The model under review builds one solid part; all positions refer to its coordinate system, in mm. Face numbers are marked on the shaded views. A direction names the side the tool comes from. Coordinates: 2 decimals unless noted, no trailing zeros. Loops run counter-clockwise (first coordinate to the right, second up) from the corner with the lowest first, then second, coordinate; pieces in that order, holes last. Notation, with made-up numbers: M 58.5,68 L 95.5,68 A7 cw 95.5,80 Z; hole C 17.25,44 d2. An arc over 180 degrees is marked long. One line per item, written item: value.
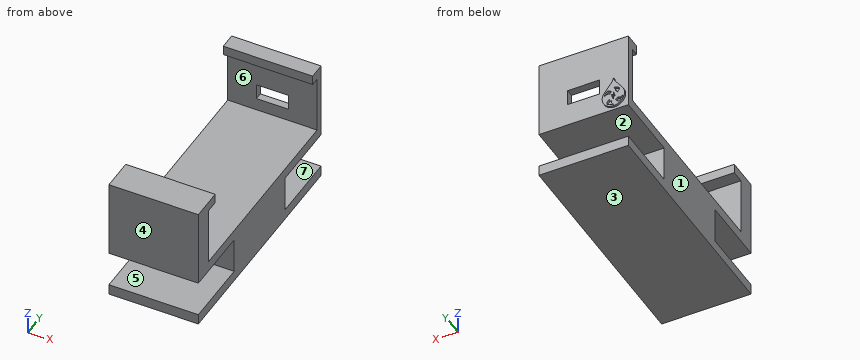
```python
from build123d import *

# Parameters (mm, degrees)
F0_W      = 42
F0_H      = 109.5
F1_DEPTH  = 5
F2_W      = 42
F2_H      = 7.5
F2_H_2    = 15
F3_DEPTH  = 32
F4_W      = 42
F4_H      = 27.5
F5_DEPTH  = 4
F6_W      = 42
F6_H      = 27.5
F7_DEPTH  = 6
F8_W      = 15
F8_H      = 7.5
F9_DEPTH  = 3.501
F10_W     = 42
F10_H     = 54.75
F11_DEPTH = 22
F12_W     = 42
F12_H     = 17
F13_DEPTH = 32
F14_W     = 42
F14_H     = 17
F15_DEPTH = 32
F17_DEPTH = 1


# Not quite as in the source:
# - a feature names something its author has since deleted; it is built from what else it names


with BuildPart() as f1:
    # F0 (on Top) → F1 (new body)
    with BuildSketch(Plane.XY):
        Rectangle(F0_W, F0_H)
    extrude(amount=F1_DEPTH)

    # F2 (on face) → F3 (join)
    with BuildSketch(Plane.XY.offset(5)):
        with Locations((0, 51)):
            Rectangle(F2_W, F2_H)
        with Locations((0, -47.25)):
            Rectangle(F2_W, F2_H_2)
    extrude(amount=F3_DEPTH)

    # F4 (on face) → F5 (cut)
    with BuildSketch(Plane.XZ.offset(-47.25)):
        with Locations((0, 18.75)):
            Rectangle(F4_W, F4_H)
    extrude(amount=-F5_DEPTH, mode=Mode.SUBTRACT)

    # F6 (on face) → F7 (cut)
    with BuildSketch(Plane(origin=(0, -39.75, 0), x_dir=(-1, 0, 0), z_dir=(0, 1, 0))):
        with Locations((0, 18.75)):
            Rectangle(F6_W, F6_H)
    extrude(amount=-F7_DEPTH, mode=Mode.SUBTRACT)

    # F8 (on face) → F9 (cut, through all)
    with BuildSketch(Plane.XZ.offset(-51.25)):
        with Locations((0, 14.75)):
            Rectangle(F8_W, F8_H)
    extrude(amount=-F9_DEPTH, mode=Mode.SUBTRACT)

    # F10 (on face) → F11 (join)
    with BuildSketch(Plane(origin=(0, 0, 0), x_dir=(1, 0, 0), z_dir=(0, 0, -1))):
        with Locations((0, -27.375)):
            Rectangle(F10_W, F10_H)
        with Locations((0, 27.375)):
            Rectangle(F10_W, F10_H)
    extrude(amount=F11_DEPTH)

    # F12 (on face) → F13 (cut)
    with BuildSketch(Plane(origin=(0, 54.75, 0), x_dir=(-1, 0, 0), z_dir=(0, 1, 0))):
        with Locations((0, -8.5)):
            Rectangle(F12_W, F12_H)
    extrude(amount=-F13_DEPTH, mode=Mode.SUBTRACT)

    # F14 (on face) → F15 (cut)
    with BuildSketch(Plane.XZ.offset(54.75)):
        with Locations((0, -8.5)):
            Rectangle(F14_W, F14_H)
    extrude(amount=-F15_DEPTH, mode=Mode.SUBTRACT)

    # F16 (on face) → F17 (join)
    with BuildSketch(Plane(origin=(0, 54.75, 0), x_dir=(-1, 0, 0), z_dir=(0, 1, 0))):
        with BuildLine():
            ThreePointArc((9.9006995692, 9.0004714316), (13.1670561221, 1.352687349), (19.7461517383, 6.4392566621))
            ThreePointArc((19.7461517383, 6.4392566621), (19.5019885984, 8.0225954525), (18.7921845523, 9.458825093))
            ThreePointArc((18.7921845523, 9.458825093), (14.575302704, 11.6944347601), (10.2883124178, 9.5963982037))
            add(Edge.make_bspline(
                [(9.9006995692, 9.0004714316), (10.0318943543, 9.2081460376), (10.1611439812, 9.4065291941), (10.2883124178, 9.5963982037)],
                knots=[0, 0, 0, 0, 0.0231761706, 0.0231761706, 0.0231761706, 0.0231761706], degree=3))
        make_face()
        with BuildLine():
            add(Edge.make_bspline(
                [(12.5148005536, 5.2476986911), (11.5117744305, 4.2282460665), (10.7037792288, 2.9078259209), (13.5031697151, 2.0462179781), (14.5618504929, 1.8354499162)],
                knots=[0, 0, 0, 0, 0.4579310006, 1, 1, 1, 1], degree=3))
            add(Edge.make_bspline(
                [(13.5659415486, 4.241716412), (12.8136013619, 4.2865276682), (12.6872834074, 4.7459304754), (12.5148005536, 5.2476986911)],
                knots=[0, 0, 0, 0, 1.4549562665, 1.4549562665, 1.4549562665, 1.4549562665], degree=3))
            add(Edge.make_bspline(
                [(14.5618504929, 1.8354499162), (14.5289066888, 1.9808173354), (13.3458541311, 2.6761364671), (13.5659415486, 4.241716412)],
                knots=[0, 0, 0, 0, 2.604218323, 2.604218323, 2.604218323, 2.604218323], degree=3))
        make_face(mode=Mode.SUBTRACT)
        Polygon((13.47238521, 7.6377728132), (14.4902859979, 7.2816363839), (14.4902859979, 9.0213598503), (15.3866174204, 5.9906424503), (14.4902859979, 6.4392566621), (14.4902859979, 4.5215808953), align=None, mode=Mode.SUBTRACT)
        with BuildLine():
            add(Edge.make_bspline(
                [(15.4229601255, 4.1801771125), (16.5064311467, 3.1538456327), (16.8590547707, 1.9119603138), (18.5636819849, 4.2745726241), (19.0433704887, 5.2473602224)],
                knots=[0, 0, 0, 0, 0.4553347248, 1, 1, 1, 1], degree=3))
            add(Edge.make_bspline(
                [(16.4662250147, 5.1379367456), (16.2283618655, 4.4227829667), (15.8584250881, 4.3158873473), (15.4229601255, 4.1801771125)],
                knots=[0, 0, 0, 0, 1.4162291989, 1.4162291989, 1.4162291989, 1.4162291989], degree=3))
            add(Edge.make_bspline(
                [(19.0433704887, 5.2473602224), (18.3244173567, 4.9723164216), (17.3367887913, 4.1913386793), (16.4662250147, 5.1379367456)],
                knots=[0, 0, 0, 0, 2.5794674433, 2.5794674433, 2.5794674433, 2.5794674433], degree=3))
        make_face(mode=Mode.SUBTRACT)
        with BuildLine():
            add(Edge.make_bspline(
                [(13.5878011524, 9.0213598503), (13.0643112241, 9.5784787958), (11.4580836083, 10.9555165738), (10.5407517819, 8.58324464), (10.0999996066, 7.6000010595)],
                knots=[0, 0, 0, 0, 0.4589082861, 1, 1, 1, 1], degree=3))
            add(Edge.make_bspline(
                [(12.7311412425, 7.7330306741), (12.9425972845, 8.4564324625), (13.1576102672, 8.8697590463), (13.5878011524, 9.0213598503)],
                knots=[0, 0, 0, 0, 1.5471451992, 1.5471451992, 1.5471451992, 1.5471451992], degree=3))
            add(Edge.make_bspline(
                [(10.0999996066, 7.6000010595), (10.8170407506, 7.9740767086), (12.6145526151, 8.968960396), (12.7311412425, 7.7330306741)],
                knots=[0, 0, 0, 0, 2.5509056967, 2.5509056967, 2.5509056967, 2.5509056967], degree=3))
        make_face(mode=Mode.SUBTRACT)
        with BuildLine():
            add(Edge.make_bspline(
                [(16.3422210337, 7.7180123234), (17.2475090665, 8.9627835512), (18.0662711639, 9.9191930916), (15.3852159818, 10.9699756355), (14.4902859979, 10.9392784796)],
                knots=[0, 0, 0, 0, 0.4716209514, 1, 1, 1, 1], degree=3))
            add(Edge.make_bspline(
                [(15.403256887, 9.0213598503), (15.9476549795, 8.7934285242), (16.1248632097, 8.3395995036), (16.3422210337, 7.7180123234)],
                knots=[0, 0, 0, 0, 1.6063525282, 1.6063525282, 1.6063525282, 1.6063525282], degree=3))
            add(Edge.make_bspline(
                [(14.4902859979, 10.9392784796), (15.2978175145, 10.325451744), (15.8282139034, 9.1764941327), (15.403256887, 9.0213598503)],
                knots=[0, 0, 0, 0, 2.1241298719, 2.1241298719, 2.1241298719, 2.1241298719], degree=3))
        make_face(mode=Mode.SUBTRACT)
        with BuildLine():
            ThreePointArc((10.2883124178, 9.5963982037), (14.575302704, 11.6944347601), (18.7921845523, 9.458825093))
            add(Edge.make_bspline(
                [(10.2883124178, 9.5963982037), (12.0270262465, 12.1923872829), (14.0912584145, 13.7285191545), (14.5502114191, 17.0414015202), (15.1068634627, 13.6426153488), (16.9710466455, 12.3841964531), (18.7921845523, 9.458825093)],
                knots=[0.0231761706, 0.0231761706, 0.0231761706, 0.0231761706, 0.3400529794, 0.5078220439, 0.6757544935, 1, 1, 1, 1], degree=3))
        make_face()
        with BuildLine():
            ThreePointArc((10.2883124178, 9.5963982037), (10.0844189973, 9.3049957736), (9.9006995692, 9.0004714316))
            add(Edge.make_bspline(
                [(9.9006995692, 9.0004714316), (10.0318943543, 9.2081460376), (10.1611439812, 9.4065291941), (10.2883124178, 9.5963982037)],
                knots=[0, 0, 0, 0, 0.0231761706, 0.0231761706, 0.0231761706, 0.0231761706], degree=3))
        make_face()
    extrude(amount=F17_DEPTH)


solid = f1.part
```
(1) Add section A-A on y = -26.5. State the section outline as (x, z) points.
Checks:
outline: M -21,-22 L 21,-22 L 21,-17 L -21,-17 Z; M -21,0 L 21,0 L 21,5 L -21,5 Z
(2) Draft analysis for pull direction Z (two halves, no side actions). For the marked faces 1, 2 and 3, state which applies: pulls with the +Z half, pulls with the -Z half, needs draft (parallel to the pull), parting line crosses it, or undercut.
Checks:
face 1: needs draft
face 2: undercut
face 3: pulls with the -Z half
(3) Add section D-D on y = -44.5. State the section outline as (x, z) points, then the cut area to 3 significant figures.
Checks:
outline: M -21,-22 L 21,-22 L 21,-17 L -21,-17 Z; M -21,0 L 21,0 L 21,5 L -21,5 Z; M -21,32.5 L 21,32.5 L 21,37 L -21,37 Z
area: 609 mm^2
(4) Add section B-B on z = 22.5. State the section outline as (x, y) points.
Checks:
outline: M -21,-54.75 L 21,-54.75 L 21,-45.75 L -21,-45.75 Z; M -21,51.25 L 21,51.25 L 21,54.75 L -21,54.75 Z
(5) To check wall thickness, follow L1, parallel to Y at x = -13, z = 17.5; L2, parallel to Z at x = 5, y = -28; L3, parallel to Y at x = 7.5, z = -12.5. State the ranges of each line that lie inside material, in increasing order. Write a range as [from, to].
Checks:
L1: [-54.75, -45.75], [51.25, 54.75]
L2: [-22, -17], [0, 5]
L3: [-22.75, 22.75]
(6) Add section C-C on x = -3. State the section outline as (y, z) points, then the cut area to 3 significant figures.
Checks:
outline: M -54.75,-22 L 54.75,-22 L 54.75,-17 L 22.75,-17 L 22.75,0 L 54.75,0 L 54.75,11 L 51.25,11 L 51.25,5 L -45.75,5 L -45.75,32.5 L -39.75,32.5 L -39.75,37 L -54.75,37 L -54.75,0 L -22.75,0 L -22.75,-17 L -54.75,-17 Z; M 47.25,32.5 L 51.25,32.5 L 51.25,18.5 L 54.75,18.5 L 54.75,37 L 47.25,37 Z
area: 2,290 mm^2
(7) Tool access review of the marked faces 4, 5, 6 and 7: name each direction out of +Z, -Z, +X, -X, +Y, -Y from which nothing blocks a thin tool from reaching the whole face with its end or side.
Checks:
face 4: +Z, -Z, +X, -X, -Y
face 5: +X, -X, -Y
face 6: +X, -X
face 7: +X, -X, +Y
(8) Insertion check: pin 1 Ø8 at (x, z) = (-1.5, 19.5) entering from +Y; pin 2 Ø12 at (y, z) = (-42, -8.5) entering from -X; pin 3 Ø4 at (x, z) = (12.5, -9.5) entering from +Y; pin 4 Ø6 at (x, y) = (7, -19) entering from +Z. Each pin has a flat end and moves straight along its axis. Give the tip position at first contact, or say it passes through.
Checks:
pin 1: y = 54.75
pin 2: through
pin 3: y = 22.75
pin 4: z = 5
